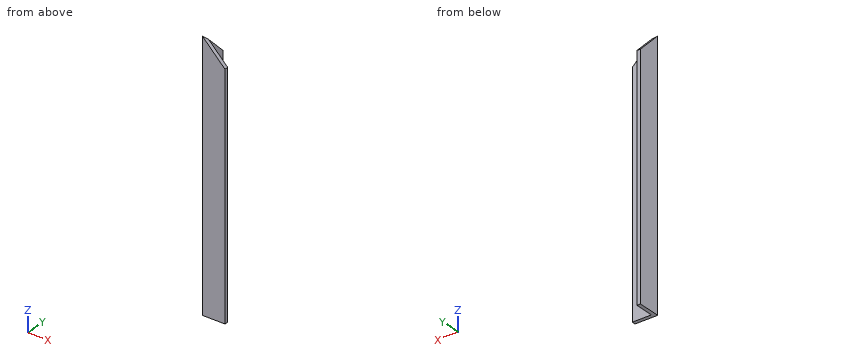
```python
from build123d import *

# Parameters (mm, degrees)
F1_DEPTH = 570
F3_DEPTH = 8
F5_DEPTH = 8


with BuildPart() as f1:
    # F0 (on Top) → F1 (new body)
    with BuildSketch(Plane.XY):
        Polygon((0, 50), (0, 0), (50, 0), (50, 8), (8, 8), (8, 50), align=None)
    extrude(amount=F1_DEPTH)

    # F2 (on face) → F3 (cut, through all)
    with BuildSketch(Plane.XZ):
        Polygon((50, 570), (0, 570), (50, 520), align=None)
    extrude(amount=-F3_DEPTH, mode=Mode.SUBTRACT)

    # F4 (on face) → F5 (cut, through all)
    with BuildSketch(Plane(origin=(0, 0, 0), x_dir=(0, -1, 0), z_dir=(-1, 0, 0))):
        Polygon((-50, 520), (0, 570), (-8, 570), (-50, 570), align=None)
    extrude(amount=-F5_DEPTH, mode=Mode.SUBTRACT)


solid = f1.part
```
Can you work these out from the model? Positions are in its coordinate system, mm. Round coordinates to 2 decimals unless told otherwise and drop trailing zeros. Loops run counter-clockwise (first coordinate to the right, second up) from the corner with the lowest first, then second, coordinate; pieces in that order, holes last. Notation, with made-up numbers: M 79.5,-14.5 L 113.5,-14.5 A27 ccw 113.5,20.5 Z; hole C 83.25,8 d1. An arc over 180 degrees is marked long. Answer in a Markdown table with one row per item.
1. I'm going to push flat-ended pins straight in: pin 1 Ø6 at (x, z) = (25, 389.5) entering from +Y; pin 2 Ø8 at (y, z) = (38.5, 389) entering from -X. Where does each tip first touch, or does it pass through?
Established:
| item | result |
|---|---|
| pin 1 | y = 8 |
| pin 2 | x = 0 |
2. If we section it at C-C, the plane y = 27: Please give me the cut outline in (x, z), plus the area to 3 significant figures.
Established:
| item | result |
|---|---|
| outline | M 0,0 L 8,0 L 8,543 L 0,543 Z |
| area | 4,340 mm² |
3. If we section it at B-B, the plane x = 42: Please give me the cut outline in (y, z).
Established:
| item | result |
|---|---|
| outline | M 0,0 L 8,0 L 8,528 L 0,528 Z |
4. If we section it at D-D, the plane z = 531: Please give me the cut outline in (x, y).
Established:
| item | result |
|---|---|
| outline | M 0,0 L 39,0 L 39,8 L 8,8 L 8,39 L 0,39 Z |
5. Please list where these lines run through material, in increasing order: line 1 (X direction, y = 15, z = 507.5); line 2 (X direction, y = 2, z = 535). Write a range as from..to.
Established:
| item | result |
|---|---|
| line 1 | 0..8 |
| line 2 | 0..35 |
6. If we section it at A-A, the plane z = 267: Please give me the cut outline in (x, y).
Established:
| item | result |
|---|---|
| outline | M 0,0 L 50,0 L 50,8 L 8,8 L 8,50 L 0,50 Z |
